Autodesk Inventor part; units mm, degrees
ref_plane "YZ Plane" through (0, 0, 0) normal (1, 0, 0) x (0, 1, 0)
ref_plane "XZ Plane" through (0, 0, 0) normal (0, 1, 0) x (-1, 0, 0)
ref_plane "XY Plane" through (0, 0, 0) normal (0, 0, 1) x (1, 0, 0)
sketch "Sketch1" plane through (0, 0, 0) normal (0, 1, 0) x (-1, 0, 0)
  line L0 (0, 0) -> (1219.2, 0)
  line L1 (1219.2, 0) -> (1219.2, -304.8)
  line L2 (1219.2, -304.8) -> (0, -304.8)
  line L3 (0, -304.8) -> (0, 0)
  dimension "d0" = 1219.2
  dimension "d1" = 304.8
extrude "Extrusion1" add sketch "Sketch1" along normal blind 2.54
sketch "Sketch2" plane through (0, 2.54, 0) normal (0, 1, 0) x (1, 0, 0)
  line L0 (-622.3, 279.4) -> (-596.9, 279.4)
  line L1 (-596.9, 279.4) -> (-596.9, 25.4)
  line L2 (-596.9, 25.4) -> (-622.3, 25.4)
  line L3 (-622.3, 25.4) -> (-622.3, 279.4)
  line L4 (-609.6, 791.1574) -> (-609.6, -567.1744) construction
  line L5 (0, 0) -> (0, 304.8)
  line L6 (0, 304.8) -> (-1219.2, 304.8)
  dimension "d4" = 254
  dimension "d5" = 25.4
  dimension "d6" = 609.6
  dimension "d7" = 12.7
  dimension "d8" = 25.4
extrude "Extrusion2" add sketch "Sketch2" along normal blind 0.254
equation "\"d7\" = 0.5 * d5"
equation "\"d8\" = d5"
properties part number "black_mid_empty"
For this review, take the finished solid that the model builds, in its own axes (mm). Coordinates: 2 decimals unless noted, no trailing zeros. Write each loop counter-clockwise with the first axis right and the second up, starting at its lowest first coordinate (ties: lowest second). Pieces come first, ordered by that corner, then holes. Notation, with made-up numbers: (11, 63.5) - (55, 63.5) arc R16 cw to (55, 75.5) - close; hole circle Ø11 at (87, -3). An arc over 180 degrees is marked (long way). Put each result on its own line as item: value.
1. Wall thickness on probe 1 along Y at (x, z) = (-238, -270.5); probe 2 along X at (y, z) = (2.6, -60.5): over which ranges is each line inside the solid? List them lowest first.
Values found:
probe 1: 0 to 2.54
probe 2: -622.3 to -596.9
2. Add section A-A, the plane z = -129.5. Give the boundary of the cut face in (x, y).
Values found:
outline: (-1219.2, 0) - (0, 0) - (0, 2.54) - (-596.9, 2.54) - (-596.9, 2.79) - (-622.3, 2.79) - (-622.3, 2.54) - (-1219.2, 2.54) - close
3. For pin 1 (6 mm diameter, centred on x = -847, z = -230.5, fed in from -Y); pin 2 (12 mm diameter, centred on x = -722, z = -252, fed in from +Y), all flat-tipped, find the tip position at first contact; note any pin that passes through.
Values found:
pin 1: y = 0
pin 2: y = 2.54
4. Add section B-B, the plane x = -470. Give the boundary of the cut face in (y, z).
Values found:
outline: (0, -304.8) - (2.54, -304.8) - (2.54, 0) - (0, 0) - close
